Can you work these out from the model? Positions are in its coordinate system, mm. A direction names the side the tool comes from. Coordinates: 2 decimals unless noted, no trailing zeros. Order: outer loops, then holes, each group sorted by start corner. A loop starts at its lowest first (then second) coordinate and runs counter-clockwise, first axis right, second up. Notation, with made-up numbers: (35.25, 20.5) -> (42.25, 20.5) arc R34 ccw to (42.25, 55.5) -> close; hole circle Ø1 at (-40, -18). An arc over 180 degrees is marked (long way). Answer in a Markdown table with one row per item. Add a question column.
1. Imagine slicing it at A-A on y = -9.5. Write out the boundary of the cut face in (x, z), plus the area to 3 significant figures.
2. Imagine slicing it at B-B on x = -1.75. State how many separate pieces and enclosed holes the cut face has, plus the area to 3 significant figures.
3. We'd pull the mould along Y, two halves only. Please class faces 4 (the face through (-2.292, -16, 1)), 5 (the face through (-0.469, -10, 1)), 6 (the face through (-0.516, 4.973, 1.708)), 7 (the face through (-1, -11, 2)): pulls with the +Y half, pulls with the -Y half, needs draft (parallel to the pull), parting line crosses it, or undercut.
4. If I drill on line 1 along Y through (x, z) = (4, 2.1); line 2 along Y through (x, z) = (0, 1.1); line 3 along Y through (x, z) = (-0.25, 0.7), over which ranges is the centre line in solid material (lowest first)? Write a range as [from, to].
5. On a 3-axis mill with a long thin cutter (end or side, diameter ignored), from which of +Z, -Z, +X, -X, +Y, -Y can I reach the whole of each face in a straight line? I mean faces 1 (the face through (3, -0.5, 1)), 2 (the face through (-4.4, -17.43, 1.01)), 3 (the face through (0, -6.052, 1)). Say none if no direction works.
from build123d import *

# Parameters (mm, degrees)
F1_DEPTH     = 3
F2_DEPTH     = 2
F3_R         = 2
F4_T1_DEPTH  = 16.75
F4_T3_DEPTH  = 6
F4_T5_DEPTH  = 16
F4_T10_DEPTH = 16.75
F4_S11_R     = 5
F4_T12_DEPTH = 10
F4_T14_ANGLE = 359.64
F4_T18_DEPTH = 19.75
F4_S19_R     = 5
F4_T20_DEPTH = 11
F4_T22_ANGLE = 90
F4_T24_ANGLE = 90
F4_T26_ANGLE = 90
F4_T28_ANGLE = 180
F4_T30_ANGLE = 90


# Not quite as in the source:
# - a fillet or chamfer that OpenCascade refuses, or shapes differently, is made with other operations: its cross-section is extruded or revolved along the edge and cut away or added


with BuildPart() as f1:
    # F0 (on Top) → F1 (new body)
    with BuildSketch(Plane.XY):
        with BuildLine():
            Line((2, 0), (5, 0))
            ThreePointArc((5, 0), (0, 5), (-5, 0))
            ThreePointArc((-5, 0), (-0.2503138753, -4.9937303656), (4.9749371855, -0.5))
            Line((4.9749371855, -0.5), (1.9364916731, -0.5))
            ThreePointArc((1.9364916731, -0.5), (-1.9840593925, 0.252008585), (2, 0))
        make_face()
    extrude(amount=F1_DEPTH)

    # F0 (on Top) → F2 (join)
    with BuildSketch(Plane.XY):
        with BuildLine():
            ThreePointArc((4.9749371855, -0.5), (-0.2503138753, -4.9937303656), (-5, 0))
            Line((-5, 0), (-5, -18))
            Line((-5, -18), (5, -18))
            Line((5, -18), (5, -0.5))
            Line((5, -0.5), (4.9749371855, -0.5))
        make_face()
        with BuildLine():
            add(Edge.make_bspline(
                [(0.578588878, -15.5900442691), (-0.0559597331, -16.3174748247), (-1.2990152887, -16.3174748247)],
                knots=[0, 0, 0, 1, 1, 1], degree=2))
            add(Edge.make_bspline(
                [(-1.2990152887, -16.3174748247), (-1.8684597331, -16.3174748247), (-2.2920708442, -16.197683158)],
                knots=[0, 0, 0, 1, 1, 1], degree=2))
            Line((-2.2920708442, -16.197683158), (-2.2920708442, -14.7983776025))
            add(Edge.make_bspline(
                [(-2.2920708442, -14.7983776025), (-1.8580430665, -14.9060164914), (-1.5004041776, -14.9060164914)],
                knots=[0, 0, 0, 1, 1, 1], degree=2))
            add(Edge.make_bspline(
                [(-1.5004041776, -14.9060164914), (-0.9465847331, -14.9060164914), (-0.7078694553, -14.5613984358)],
                knots=[0, 0, 0, 1, 1, 1], degree=2))
            add(Edge.make_bspline(
                [(-0.7078694553, -14.5613984358), (-0.4691541776, -14.2167803802), (-0.4691541776, -13.4841414914)],
                knots=[0, 0, 0, 1, 1, 1], degree=2))
            Line((-0.4691541776, -13.4841414914), (-0.4691541776, -6.0518498247))
            Line((-0.4691541776, -6.0518498247), (1.2131374891, -6.0518498247))
            Line((1.2131374891, -6.0518498247), (1.2131374891, -13.4737248247))
            add(Edge.make_bspline(
                [(1.2131374891, -13.4737248247), (1.2131374891, -14.8626137136), (0.578588878, -15.5900442691)],
                knots=[0, 0, 0, 1, 1, 1], degree=2))
        make_face(mode=Mode.SUBTRACT)
    extrude(amount=F2_DEPTH)

    # F3
    f3_edges = [f1.edges().sort_by_distance(p)[0] for p in [
        (-5, -18, 1),
        (5, -18, 1),
    ]]
    fillet(f3_edges, radius=F3_R)

    # F4: fillet of radius 0.5 on 12 edges, made by hand

    # F4_s2 → F4_t1 (cut)
    with BuildSketch(Plane.XZ.offset(-0.75)):
        with BuildLine():
            ThreePointArc((5, 0.5), (4.8535533906, 0.1464466094), (4.5, 0))
            Line((4.5, 0), (5, 0))
            Line((5, 0), (5, 0.5))
        make_face()
    extrude(amount=F4_T1_DEPTH, mode=Mode.SUBTRACT)

    # F4_s4 → F4_t3 (cut)
    with BuildSketch(Plane.YZ.offset(-3)):
        with BuildLine():
            ThreePointArc((-17.5, 2), (-17.8535533906, 1.8535533906), (-18, 1.5))
            Line((-18, 1.5), (-18, 2))
            Line((-18, 2), (-17.5, 2))
        make_face()
        with BuildLine():
            ThreePointArc((-18, 0.5), (-17.8535533906, 0.1464466094), (-17.5, 0))
            Line((-17.5, 0), (-18, 0))
            Line((-18, 0), (-18, 0.5))
        make_face()
    extrude(amount=F4_T3_DEPTH, mode=Mode.SUBTRACT)

    # F4_s6 → F4_t5 (cut)
    with BuildSketch(Plane.XZ):
        with BuildLine():
            ThreePointArc((-5, 0.5), (-4.8535533906, 0.1464466094), (-4.5, 0))
            Line((-4.5, 0), (-5, 0))
            Line((-5, 0), (-5, 0.5))
        make_face()
    extrude(amount=F4_T5_DEPTH, mode=Mode.SUBTRACT)


with BuildPart() as f4_tool8:
    # F4_s9 → F4_t10 (new body)
    with BuildSketch(Plane.XZ.offset(16)):
        with BuildLine():
            ThreePointArc((4.5, 2), (4.8535533906, 1.8535533906), (5, 1.5))
            Line((5, 1.5), (5, 2))
            Line((5, 2), (4.5, 2))
        make_face()
    extrude(amount=-F4_T10_DEPTH)

    # F4_s11 → F4_t12 (cut, symmetric)
    with BuildSketch(Plane.XY.offset(1.8)):
        Circle(F4_S11_R)
    extrude(amount=F4_T12_DEPTH, both=True, mode=Mode.SUBTRACT)


with BuildPart() as f1_1:
    add(f1.part)

    # F4_t7: cut F4_tool8
    add(f4_tool8.part, mode=Mode.SUBTRACT)

    # F4_s13 → F4_t14 (revolve, cut)
    with BuildSketch(Plane(origin=(0, 0, 0), x_dir=(0, 0, 1), z_dir=(0.0532001762, 0.9985838679, 0))):
        with BuildLine():
            ThreePointArc((2.5, 5), (2.8535533906, 4.8535533906), (3, 4.5))
            Line((3, 4.5), (3, 5))
            Line((3, 5), (2.5, 5))
        make_face()
    revolve(axis=Axis((0, 0, 3), (0, 0, -1)), revolution_arc=F4_T14_ANGLE, mode=Mode.SUBTRACT)


with BuildPart() as f4_tool16:
    # F4_s17 → F4_t18 (new body)
    with BuildSketch(Plane.XZ.offset(-3.75)):
        with BuildLine():
            ThreePointArc((-4.5, 2), (-4.8535533906, 1.8535533906), (-5, 1.5))
            Line((-5, 1.5), (-5, 2))
            Line((-5, 2), (-4.5, 2))
        make_face()
    extrude(amount=F4_T18_DEPTH)

    # F4_s19 → F4_t20 (cut, symmetric)
    with BuildSketch(Plane.XY.offset(1.8)):
        Circle(F4_S19_R)
    extrude(amount=F4_T20_DEPTH, both=True, mode=Mode.SUBTRACT)


with BuildPart() as f1_2:
    add(f1_1.part)

    # F4_t15: cut F4_tool16
    add(f4_tool16.part, mode=Mode.SUBTRACT)

    # F4_s21 → F4_t22 (revolve, cut)
    with BuildSketch(Plane.YZ.offset(-3)):
        with BuildLine():
            ThreePointArc((-17.5, 2), (-17.8535533906, 1.8535533906), (-18, 1.5))
            Line((-18, 1.5), (-18, 2))
            Line((-18, 2), (-17.5, 2))
        make_face()
    revolve(axis=Axis((-3, -16, 2), (0, 0, -1)), revolution_arc=F4_T22_ANGLE, mode=Mode.SUBTRACT)

    # F4_s23 → F4_t24 (revolve, cut)
    with BuildSketch(Plane.YZ.offset(3)):
        with BuildLine():
            ThreePointArc((-17.5, 2), (-17.8535533906, 1.8535533906), (-18, 1.5))
            Line((-18, 1.5), (-18, 2))
            Line((-18, 2), (-17.5, 2))
        make_face()
    revolve(axis=Axis((3, -16, 2), (0, 0, 1)), revolution_arc=F4_T24_ANGLE, mode=Mode.SUBTRACT)

    # F4_s25 → F4_t26 (revolve, cut)
    with BuildSketch(Plane.YZ.offset(-3)):
        with BuildLine():
            ThreePointArc((-18, 0.5), (-17.8535533906, 0.1464466094), (-17.5, 0))
            Line((-17.5, 0), (-18, 0))
            Line((-18, 0), (-18, 0.5))
        make_face()
    revolve(axis=Axis((-3, -16, 0), (0, 0, -1)), revolution_arc=F4_T26_ANGLE, mode=Mode.SUBTRACT)

    # F4_s27 → F4_t28 (revolve, cut)
    with BuildSketch(Plane.XZ):
        with BuildLine():
            ThreePointArc((5, 0.5), (4.8535533906, 0.1464466094), (4.5, 0))
            Line((4.5, 0), (5, 0))
            Line((5, 0), (5, 0.5))
        make_face()
    revolve(axis=Axis((0, 0, 0), (0, 0, 1)), revolution_arc=F4_T28_ANGLE, mode=Mode.SUBTRACT)

    # F4_s29 → F4_t30 (revolve, cut)
    with BuildSketch(Plane.YZ.offset(3)):
        with BuildLine():
            ThreePointArc((-18, 0.5), (-17.8535533906, 0.1464466094), (-17.5, 0))
            Line((-17.5, 0), (-18, 0))
            Line((-18, 0), (-18, 0.5))
        make_face()
    revolve(axis=Axis((3, -16, 0), (0, 0, 1)), revolution_arc=F4_T30_ANGLE, mode=Mode.SUBTRACT)


solid = f1_2.part
Answers follow:
| question | item | result |
|---|---|---|
| 1 | outline | (-5, 0.5) arc R0.5 ccw to (-4.5, 0) -> (-0.47, 0) -> (-0.47, 2) -> (-4.5, 2) arc R0.5 ccw to (-5, 1.5) -> close; (1.21, 0) -> (4.5, 0) arc R0.5 ccw to (5, 0.5) -> (5, 1.5) arc R0.5 ccw to (4.5, 2) -> (1.21, 2) -> close |
| 1 | area | 16.4 mm² |
| 2 | separate pieces | 3 |
| 2 | enclosed holes | 0 |
| 2 | area | 45.8 mm² |
| 3 | face 4 | undercut |
| 3 | face 5 | undercut |
| 3 | face 6 | parting line crosses it |
| 3 | face 7 | needs draft |
| 4 | line 1 | y = [-3, -0.5], [0, 3] |
| 4 | line 2 | y = [-18, -16.04], [-6.05, -2], [2, 5] |
| 4 | line 3 | y = [-18, -16.15], [-6.05, -1.98], [1.98, 4.99] |
| 5 | face 1 | +Z, -Z, +X |
| 5 | face 2 | +Z, -Z, -X, -Y |
| 5 | face 3 | +Z, -Z |
